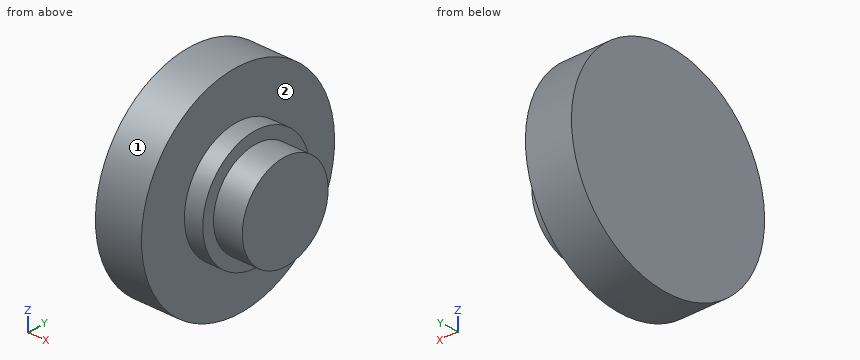
```python
from build123d import *

# Parameters (mm, degrees)
F0_W = 2.5
F0_H = 4


with BuildPart() as f1:
    # F0 (on Front) → F1 (revolve)
    with BuildSketch(Plane.XZ):
        Polygon((-7.152688, 5), (-7.152688, 0), (-5.552688, 0), (-5.552688, 4), (-5.552688, 5), align=None)
        Polygon((-11.152688, 0), (-7.152688, 0), (-7.152688, 5), (-7.152688, 9), (-11.152688, 9), (-11.152688, 8.198828), align=None)
        with Locations((-4.302688, 2)):
            Rectangle(F0_W, F0_H)
    revolve(axis=Axis((-2.808182, 0, 0), (1, 0, 0)))


solid = f1.part
```
For this review, take the finished solid that the model builds, in its own axes (mm). Face numbers are marked on the shaded views. A direction names the side the tool comes from. Coordinates: 2 decimals unless noted, no trailing zeros. Write each loop counter-clockwise with the first axis right and the second up, starting at its lowest first coordinate (ties: lowest second). Pieces come first, ordered by that corner, then holes. Notation, with made-up numbers: (49.25, 81) - (96.25, 81) arc R13 cw to (96.25, 104) - close; hole circle Ø5 at (35.5, -15.75). An arc over 180 degrees is marked (long way). Answer in a Markdown table with one row per item. Add a question column.
Q1. Tool access review of the marked faces 1 and 2: name each direction out of +Z, -Z, +X, -X, +Y, -Y from which nothing blocks a thin tool from reaching the whole face with its end or side.
Q2. For probe 1 along X at (y, z) = (-2, 4.5); probe 2 along X at (y, z) = (2.75, -6); probe 3 along Z at (x, y) = (-4.5, -2.5), list the stretches that pass through material, from the lowest coordinate up.
Q3. For P1, Ø1, axis at x = -7.5, y = -1, coming from the +Z side; P2, Ø2, axis at x = -4.5, z = -7, coming from the -Y side; P3, Ø4, axis at x = -7, z = 2.5, coming from the -Y side; P4, Ø3, axis at x = -4.5, y = 2, coming from the +Z side, all flat-tipped, find the tip position at first contact; note any pin that passes through.
Q4. We need section A-A, the plane y = 0. State the section outline as (x, z) points.
Q5. We need section D-D, the plane y = 5.25. State the section outline as (x, z) points.
Q6. We need section C-C, the plane x = -9. State the section outline as (y, z) points, and give its area (3 significant figures).
Answer list:
| question | item | result |
|---|---|---|
| 1 | face 1 | +X, -X |
| 1 | face 2 | +X |
| 2 | probe 1 | x = -11.15 to -5.55 |
| 2 | probe 2 | x = -11.15 to -7.15 |
| 2 | probe 3 | z = -3.12 to 3.12 |
| 3 | P1 | stops at z = 8.99 |
| 3 | P2 | passes through |
| 3 | P3 | stops at y = -8.99 |
| 3 | P4 | stops at z = 4.91 |
| 4 | outline | (-11.15, -9) - (-7.15, -9) - (-7.15, -5) - (-5.55, -5) - (-5.55, -4) - (-3.05, -4) - (-3.05, 4) - (-5.55, 4) - (-5.55, 5) - (-7.15, 5) - (-7.15, 9) - (-11.15, 9) - close |
| 5 | outline | (-11.15, -7.31) - (-7.15, -7.31) - (-7.15, 7.31) - (-11.15, 7.31) - close |
| 6 | outline | circle Ø18 at (0, 0) |
| 6 | area | 254 mm2 |
